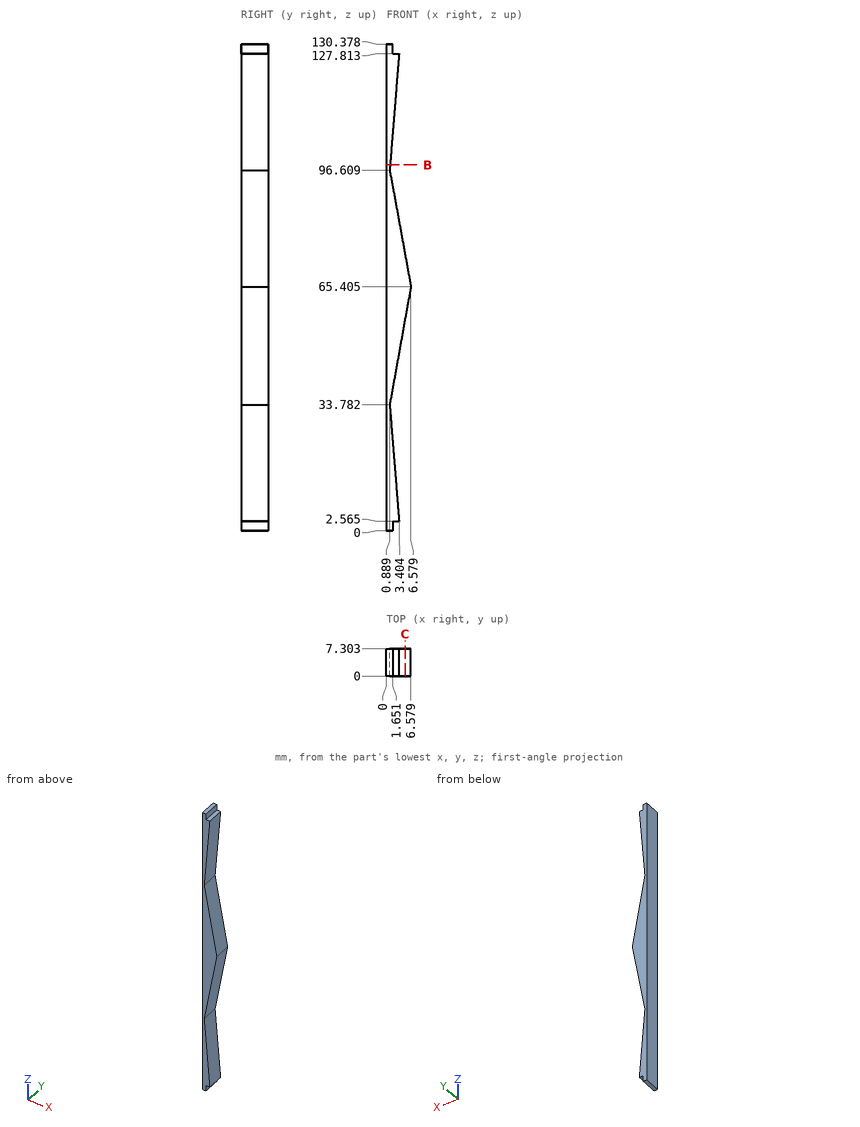
Here's the drawing with two shaded views (mm, measured from the low corner). I have some questions. Round coordinates to 2 decimals unless told otherwise and drop trailing zeros. Write each loop counter-clockwise with the first axis right and the second up, starting at its lowest first coordinate (ties: lowest second). Pieces come first, ordered by that corner, then holes. Notation, with made-up numbers: M 45,36.25 L 88,36.25 A7 cw 88,46.25 Z; hole C 58.25,40 d6. An arc over 180 degrees is marked long. Answer in a Markdown table with one row per item. Add a question column.
Q1. Will these pins go through, and if not, where does the flat tip stop? pin 1 Ø1.9 at (x, y) = (2, 3) entering from +Z; pin 2 Ø0.8 at (y, z) = (2.5, 129) entering from +X; pin 3 Ø3 at (y, z) = (1, 63) entering from +X (1 decimal); pin 4 Ø4 at (y, z) = (4, 101.5) entering from +X.
Q2. Imagine slicing it at C-C (x = 5). Please give me the cut outline in (y, z), then the cut area to 3 significant figures.
Q3. Imagine slicing it at B-B (z = 98). Please give me the cut outline in (x, y).
Q4. If I drill on line 1 (X direction, y = 2, z = 19.5); line 2 (X direction, y = 6.5, z = 85.5) (1 decimal), over which ranges is the centre line in solid material (lowest first)? Write a range as from..to.
Values:
| question | item | result |
|---|---|---|
| 1 | pin 1 | z = 130.38 |
| 1 | pin 2 | x = 1.65 |
| 1 | pin 3 | x = 6.4 |
| 1 | pin 4 | x = 1.44 |
| 2 | outline | M 0,56.63 L 7.3,56.63 L 7.3,74.06 L 0,74.06 Z |
| 2 | area | 127 mm^2 |
| 3 | outline | M 0,0 L 1,0 L 1,7.3 L 0,7.3 Z |
| 4 | line 1 | 0..2.04 |
| 4 | line 2 | 0..2.9 |
